Drawing for the job (mm, zero at the part's lowest x, y, z). A direction names the side the tool comes from. Round coordinates to 2 decimals unless told otherwise and drop trailing zeros. Write each loop counter-clockwise with the first axis right and the second up, starting at its lowest first coordinate (ties: lowest second). Pieces come first, ordered by that corner, then holes. Notation, with made-up numbers: M -33.75,39 L 16.25,39 A15 ccw 16.25,51 Z; hole C 47.25,47.5 d2. An arc over 180 degrees is marked long. Use a Markdown table: item, result. Add a question column.
1) Slice it at B-B on y = 1.25. Write the cut outline in (x, z), plus the area to 3 significant figures.
2) Slice it at C-C on z = 6.5. Write the cut outline in (x, y), plus the area to 3 significant figures.
3) Slice it at A-A on z = 2.75. Write the cut outline in (x, y), plus the area to 3 significant figures.
4) Wall check: probe 1 along X at (y, z) = (2, 4.75); probe 2 along Y at (x, z) = (14, 8). Give the ranges that are in metal, low to high.
5) Slice it at D-D on x = 13. Write the cut outline in (y, z).
6) Which spindle directions (+Z, -Z, +X, -X, +Y, -Y) get a long thin tool onto all of the face, cutting with end or side? Do the marked faces 1 and 2. Say none if no direction does.
7) Drop flat-ended pins along their axis: P1, Ø2, axis at x = 7, z = 1, coming from the +Y side; P2, Ø3, axis at x = 11.5, y = 3.5, coming from the +Z side (3 decimals); P3, Ø1.1, axis at x = 13.5, y = 0.5, coming from the -Z side. Give the stop position or say it passes through.
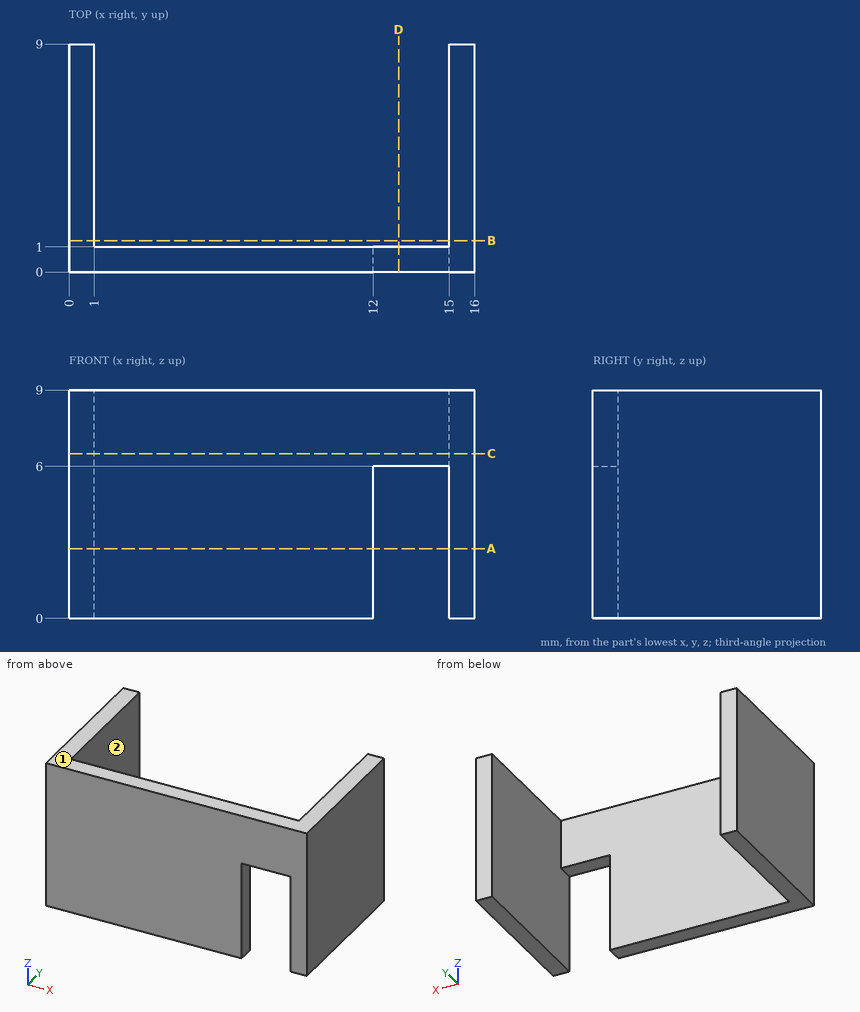
Entries:
| question | item | result |
|---|---|---|
| 1 | outline | M 0,0 L 1,0 L 1,9 L 0,9 Z; M 15,0 L 16,0 L 16,9 L 15,9 Z |
| 1 | area | 18.0 mm^2 |
| 2 | outline | M 0,0 L 16,0 L 16,9 L 15,9 L 15,1 L 1,1 L 1,9 L 0,9 Z |
| 2 | area | 32.0 mm^2 |
| 3 | outline | M 0,0 L 12,0 L 12,1 L 1,1 L 1,9 L 0,9 Z; M 15,0 L 16,0 L 16,9 L 15,9 Z |
| 3 | area | 29.0 mm^2 |
| 4 | probe 1 | x = 0 to 1, 15 to 16 |
| 4 | probe 2 | y = 0 to 1 |
| 5 | outline | M 0,6 L 1,6 L 1,9 L 0,9 Z |
| 6 | face 1 | +Z, +X, -X, +Y, -Y |
| 6 | face 2 | +Z, -Z, +Y |
| 7 | P1 | stops at y = 1 |
| 7 | P2 | passes through |
| 7 | P3 | stops at z = 6 |
